Input: part model. Units: mm. Frame: model coordinates. Face numbers are marked on the shaded views. A direction names the side the tool comes from. Coordinates: 2 decimals unless noted, no trailing zeros. Write each loop counter-clockwise with the first axis right and the second up, starting at its lowest first coordinate (ties: lowest second). Pieces come first, ordered by that corner, then holes.
1) Section query D-D (z = 9.5). Output: boundary loops of the cut face in (x, y).
2) Set-up query: the marked faces 1 and 2. Return all of +Z, -Z, +X, -X, +Y, -Y with unobstructed straight access to the full face (end or side cutting, diameter ignored); none if empty.
3) Section query A-A (x = 0). Output: boundary loops of the cut face in (y, z), then the cut area to 3 significant figures.
4) Section query B-B (z = -3). Output: boundary loops of the cut face in (x, y).
5) Pin query (flat end, axial travel): pin 1 Ø1 at (y, z) = (-8.5, 3) entering from +X; pin 2 Ø0.7 at (x, y) = (-6.5, -6.5) entering from +Z; pin 3 Ø1.7 at (y, z) = (-1.5, 22.5) entering from +X; pin 4 Ø12 at (x, y) = (2, -7) entering from +Z. Return the tip coordinate at first contact, or that it passes through.
6) Line query: L1, parallel to X at y = -6.25, z = 19; L2, parallel to Z at x = 5.5, y = 7.5; L3, parallel to Z at x = -0.5, y = 5.25. Output: solid intervals per line, ascending.
7) Section query C-C (y = -3). Output: boundary loops of the cut face in (x, z), then the cut area to 3 significant figures.
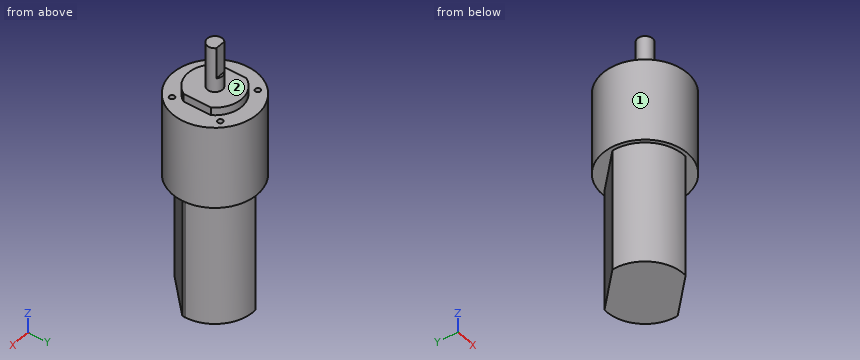
from build123d import *

# Parameters (mm, degrees)
F0_R      = 11.049
F1_DEPTH  = 21.717
F3_DEPTH  = 2.0828
F4_R      = 1.9812
F5_DEPTH  = 11.8618
F7_DEPTH  = 8.1788
F8_R      = 0.6858
F9_DEPTH  = 4.064
F11_DEPTH = 32.2072


with BuildPart() as f1:
    # F0 (on Top) → F1 (new body)
    with BuildSketch(Plane.XY):
        Circle(F0_R)
    extrude(amount=F1_DEPTH)

    # F2 (on face) → F3 (join)
    with BuildSketch(Plane.XY.offset(21.717)):
        with BuildLine():
            Line((5.9944, -3.610398), (5.9944, 3.610398))
            ThreePointArc((5.9944, 3.610398), (0, 6.9977), (-5.9944, 3.610398))
            Line((-5.9944, 3.610398), (-5.9944, -3.610398))
            ThreePointArc((-5.9944, -3.610398), (0, -6.9977), (5.9944, -3.610398))
        make_face()
    extrude(amount=F3_DEPTH)

    # F4 (on face) → F5 (join)
    with BuildSketch(Plane.XY.offset(23.7998)):
        Circle(F4_R)
    extrude(amount=F5_DEPTH)

    # F6 (on face) → F7 (cut)
    with BuildSketch(Plane.XY.offset(35.6616)):
        with BuildLine():
            ThreePointArc((1.379105, 1.4224), (0, 1.9812), (-1.379105, 1.4224))
            Line((-1.379105, 1.4224), (1.379105, 1.4224))
        make_face()
    extrude(amount=-F7_DEPTH, mode=Mode.SUBTRACT)

    # F8 (on face) → F9 (cut)
    with BuildSketch(Plane.XY.offset(21.717)):
        with Locations((-6.35, 6.35)):
            Circle(F8_R)
        with Locations((6.35, 6.35)):
            Circle(F8_R)
        with Locations((6.35, -6.35)):
            Circle(F8_R)
        with Locations((-6.35, -6.35)):
            Circle(F8_R)
    extrude(amount=-F9_DEPTH, mode=Mode.SUBTRACT)

    # F10 (on face) → F11 (join)
    with BuildSketch(Plane(origin=(0, 0, 0), x_dir=(1, 0, 0), z_dir=(0, 0, -1))):
        with BuildLine():
            ThreePointArc((-0.748756, -10.081433), (6.878466, -7.408281), (10.1092, 0))
            ThreePointArc((10.1092, 0), (10.102256, 0.374635), (10.081433, 0.748756))
            Line((10.081433, 0.748756), (0.748756, 10.081433))
            ThreePointArc((0.748756, 10.081433), (-7.148284, 7.148284), (-10.081433, -0.748756))
            Line((-10.081433, -0.748756), (-0.748756, -10.081433))
        make_face()
    extrude(amount=F11_DEPTH)


solid = f1.part
Answer:
1. outline: circle Ø22.1 at (0, 0)
2. face 1: +Z, -Z
2. face 2: +Z
3. outline: (-11.05, 0) - (-10.11, 0) - (-10.11, -32.21) - (10.11, -32.21) - (10.11, 0) - (11.05, 0) - (11.05, 21.72) - (7, 21.72) - (7, 23.8) - (1.98, 23.8) - (1.98, 27.48) - (1.42, 27.48) - (1.42, 35.66) - (-1.98, 35.66) - (-1.98, 23.8) - (-7, 23.8) - (-7, 21.72) - (-11.05, 21.72) - close
3. area: 1,200 mm2
4. outline: (-10.08, 0.75) arc R10.11 ccw to (0.75, -10.08) - (10.08, -0.75) arc R10.11 ccw to (10.11, 0) arc R10.11 ccw to (-0.75, 10.08) - close
5. pin 1: stops at x = 7.62
5. pin 2: stops at z = 17.65
5. pin 3: stops at x = 10.99
5. pin 4: stops at z = 35.66
6. L1: x = -9.11 to -7.03, -5.67 to 5.67, 7.03 to 9.11
6. L2: z = -32.21 to 21.72
6. L3: z = -32.21 to 23.8
7. outline: (-10.63, 0) - (-9.65, 0) - (-9.65, -32.21) - (7.83, -32.21) - (7.83, 0) - (10.63, 0) - (10.63, 21.72) - (5.99, 21.72) - (5.99, 23.8) - (-5.99, 23.8) - (-5.99, 21.72) - (-10.63, 21.72) - close
7. area: 1,050 mm2
